from build123d import *

# Parameters (mm, degrees)
F0_W     = 8
F0_H     = 16
F1_DEPTH = 3.2
F3_DEPTH = 1.7


# Not quite as in the source:
# - a feature names something its author has since deleted; it is built from what else it names


with BuildPart() as f1:
    # F0 (on Right) → F1 (new body)
    with BuildSketch(Plane.YZ):
        with Locations((4, 8)):
            Rectangle(F0_W, F0_H)
    extrude(amount=F1_DEPTH)

    # F2 (on face) → F3 (join)
    with BuildSketch(Plane.YZ.offset(3.2)):
        with BuildLine():
            ThreePointArc((4.0419005416, 9.7116244191), (5.7227796266, 10.4232962474), (6.4169111453, 12.1114943177))
            ThreePointArc((6.4169111453, 12.1114943177), (5.730047367, 13.7923168204), (4.0626075738, 14.5110592441))
            Line((4.0626075738, 14.5110592441), (4.0419005416, 9.7116244191))
        make_face()
        with BuildLine():
            Line((4.0419005416, 9.7116244191), (4.0626075738, 14.5110592441))
            ThreePointArc((4.0626075738, 14.5110592441), (1.6169334826, 12.1218489566), (4.0419005416, 9.7116244191))
        make_face()
        with BuildLine():
            ThreePointArc((6.4169111453, 3.9196317084), (5.7176243976, 5.6130231083), (4.0272657842, 6.3196093711))
            Line((4.0272657842, 6.3196093711), (4.0272298946, 6.3112909609))
            Line((4.0272298946, 6.3112909609), (4.0065565064, 1.5196540457))
            ThreePointArc((4.0065565064, 1.5196540457), (5.7103025452, 2.2189184561), (6.4169111453, 3.9196317084))
        make_face()
        with BuildLine():
            Line((4.0272298946, 6.3112909609), (4.0272657842, 6.3196093711))
            ThreePointArc((4.0272657842, 6.3196093711), (1.6169334826, 3.9299863473), (4.0065565064, 1.5196540457))
            Line((4.0065565064, 1.5196540457), (4.0272298946, 6.3112909609))
        make_face()
    extrude(amount=F3_DEPTH)


solid = f1.part
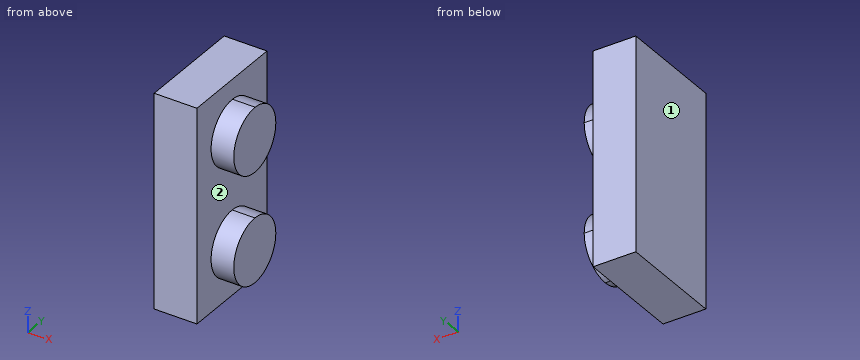
Verification items for the finished model (mm, model axes). Face numbers are marked on the shaded views. A direction names the side the tool comes from. Coordinates: 2 decimals unless noted, no trailing zeros. Write each loop counter-clockwise with the first axis right and the second up, starting at its lowest first coordinate (ties: lowest second). Pieces come first, ordered by that corner, then holes. Notation, with made-up numbers: (27, -32.5) - (68, -32.5) arc R24 cw to (68, -7.5) - close; hole circle Ø9 at (61.5, 63). An arc over 180 degrees is marked (long way). Answer as a JSON object with one key per item and string values.
(1) Cross-section at D-D on y = 5. Record the cut outline in (x, z).
Report:
{"outline": "(0, 0) - (3.2, 0) - (3.2, 1.73) - (4.9, 1.73) - (4.9, 6.11) - (3.2, 6.11) - (3.2, 9.92) - (4.9, 9.92) - (4.9, 14.3) - (3.2, 14.3) - (3.2, 16) - (0, 16) - close"}
(2) Thickness scan on line 1 along X through (y, z) = (3.75, 7.75); line 2 along Z through (x, y) = (3.9, 3); line 3 along Y through (x, z) = (3.55, 10). Record the ranges inside material, lowest first.
Report:
{"line 1": "0 to 3.2", "line 2": "1.75 to 6.09, 9.94 to 14.29", "line 3": "2.88 to 5.16"}
(3) Cross-section at B-B on y = 2. Record the cut outline in (x, z).
Report:
{"outline": "(0, 0) - (3.2, 0) - (3.2, 2.62) - (4.9, 2.62) - (4.9, 5.22) - (3.2, 5.22) - (3.2, 10.81) - (4.9, 10.81) - (4.9, 13.41) - (3.2, 13.41) - (3.2, 16) - (0, 16) - close"}
(4) Cross-section at A-A on x = 4.2. Record the cut outline in (y, z), plus the area to 3 significant figures.
Report:
{"outline": "circle Ø4.8 at (4.02, 3.92); circle Ø4.8 at (4.02, 12.11)", "area": "36.2 mm^2"}
(5) Tool access check on the marked faces 1 and 2. Record the directions out of +Z, -Z, +X, -X, +Y, -Y that give a thin tool (end or side, any length) a straight path to the whole face; none if there is none.
Report:
{"face 1": "+Z, -Z, -X, +Y, -Y", "face 2": "+X"}
(6) Cross-section at C-C on z = 2.75. Record the cut outline in (x, y).
Report:
{"outline": "(0, 0) - (3.2, 0) - (3.2, 1.92) - (4.9, 1.92) - (4.9, 6.11) - (3.2, 6.11) - (3.2, 8) - (0, 8) - close"}
